Source: CAD feature listing. Evaluate the final solid. Frame: model axes, mm. A direction names the side the tool comes from. Give positions to 0.01 mm unless a question says otherwise; leave off trailing zeros. Write each loop counter-clockwise with the first axis right and the second up, starting at its lowest first coordinate (ties: lowest second). Pieces come first, ordered by that corner, then holes. Notation, with made-up numbers: (38, 4.5) -> (74, 4.5) arc R11 cw to (74, 9.5) -> close; hole circle Ø3 at (30.5, -26). An arc over 180 degrees is marked (long way). Write item = value, one per line.
from build123d import *

# Parameters (mm, degrees)
SKETCH1_W            = 250
SKETCH1_H            = 100
BOSS_EXTRUDE1_DEPTH  = 5
SKETCH2_W            = 5
SKETCH2_H            = 100
BOSS_EXTRUDE2_DEPTH  = 50
FILLET1_R            = 20
BOSS_EXTRUDE3_START  = -250
SKETCH3_R            = 5
BOSS_EXTRUDE3_DEPTH  = 40
BOSS_EXTRUDE4_START  = 40
SKETCH3_2_R          = 5
BOSS_EXTRUDE4_DEPTH  = 40
SKETCH4_R            = 10
BOSS_EXTRUDE5_DEPTH  = 500
SKETCH6_R            = 7.5
BOSS_EXTRUDE9_DEPTH  = 5
BOSS_EXTRUDE11_START = 5
SKETCH7_R            = 7.5
BOSS_EXTRUDE11_DEPTH = 5
FILLET3_R            = 2.5


with BuildPart() as part:
    # Sketch1 → Boss-Extrude1 (new body)
    with BuildSketch(Plane(origin=(0, 0, 0), x_dir=(1, 0, 0), z_dir=(0, 1, 0))):
        Rectangle(SKETCH1_W, SKETCH1_H)
    extrude(amount=BOSS_EXTRUDE1_DEPTH)

    # Sketch2 → Boss-Extrude2 (add)
    with BuildSketch(Plane(origin=(0, 5, 0), x_dir=(1, 0, 0), z_dir=(0, 1, 0))):
        with Locations((-122.5, 0)):
            Rectangle(SKETCH2_W, SKETCH2_H)
        with Locations((122.5, 0)):
            Rectangle(SKETCH2_W, SKETCH2_H)
    extrude(amount=BOSS_EXTRUDE2_DEPTH)

    # Fillet1
    fillet1_edges = [part.edges().sort_by_distance(p)[0] for p in [
        (122.5, 55, -50),
        (122.5, 55, 50),
        (-122.5, 55, -50),
        (-122.5, 55, 50),
    ]]
    fillet(fillet1_edges, radius=FILLET1_R)

    # Sketch3 → Boss-Extrude3 (add)
    with BuildSketch(Plane.ZY.offset(125).offset(BOSS_EXTRUDE3_START)):
        with Locations((0, 27.5)):
            Circle(SKETCH3_R)
    extrude(amount=-BOSS_EXTRUDE3_DEPTH)

    # Sketch3<2> → Boss-Extrude4 (add)
    with BuildSketch(Plane.ZY.offset(125).offset(BOSS_EXTRUDE4_START)):
        with Locations((0, 27.5)):
            Circle(SKETCH3_2_R)
    extrude(amount=-BOSS_EXTRUDE4_DEPTH)

    # Sketch4 → Boss-Extrude5 (add)
    with BuildSketch(Plane(origin=(0, 0, 0), x_dir=(-1, 0, 0), z_dir=(0, -1, 0))):
        with Locations(Location((0, 0, 0), (0, 0, 270))):
            Circle(SKETCH4_R)
    extrude(amount=BOSS_EXTRUDE5_DEPTH)

    # Sketch6 → Boss-Extrude9 (add)
    with BuildSketch(Plane(origin=(165, 0, 0), x_dir=(0, 0, -1), z_dir=(1, 0, 0))):
        with Locations((0, 27.5)):
            Circle(SKETCH6_R)
    extrude(amount=BOSS_EXTRUDE9_DEPTH)

    # Sketch7 → Boss-Extrude11 (add)
    with BuildSketch(Plane.ZY.offset(165).offset(BOSS_EXTRUDE11_START)):
        with Locations(Location((0, 27.5, 0), (0, 0, 180))):
            Circle(SKETCH7_R)
    extrude(amount=-BOSS_EXTRUDE11_DEPTH)

    # Fillet3
    fillet3_edges = [part.edges().sort_by_distance(p)[0] for p in [
        (-120, 5, 0),
        (120, 5, 0),
    ]]
    fillet(fillet3_edges, radius=FILLET3_R)


solid = part.part
(1) Section query D-D (x = -104). Return loops of the section in (y, z), plus the area to 3 significant figures.
Values follow:
outline = (0, -50) -> (5, -50) -> (5, 50) -> (0, 50) -> close
area = 500 mm2
(2) Section query B-B (z = 40). Return loops of the section in (x, y).
Values follow:
outline = (-125, 0) -> (125, 0) -> (125, 52.32) -> (120, 52.32) -> (120, 7.5) arc R2.5 cw to (117.5, 5) -> (-117.5, 5) arc R2.5 cw to (-120, 7.5) -> (-120, 52.32) -> (-125, 52.32) -> close
(3) Section query C-C (y = -123). Return loops of the section in (x, z), plus the area to 3 significant figures.
Values follow:
outline = circle Ø20 at (0, 0)
area = 314 mm2
(4) Access query for faces 1 (the face through (0, -500, 0)), 2 (the face through (-145.28, 22.62, -1.08)), 3 (the face through (122.535, 48.986, 44.297)), 4 (the face through (9.76, -246.5, -2.17)), 5 (the face through (-2, 5, -1)). Directions: +Z, -Z, +X, -X, +Y, -Y. A direction counts if a zero-diameter tool reaches every point of the face in a straight line with its end or side. Return the directions, or none.
Values follow:
face_1 = +Z, -Z, +X, -X, -Y
face_2 = none
face_3 = +Z, +X, -X, +Y
face_4 = -Y
face_5 = +Z, -Z, +Y
(5) Pull-direction query (X, two-part tool) for faces 6 (the face through (-170, 27, 0)), 7 (the face through (120, 31, 1)), 8 (the face through (-2, 0, -12)); classes: pulls with the +X half, pulls with the -X half, needs draft (parallel to the pull), parting line crosses it, or undercut.
Values follow:
face_6 = pulls with the -X half
face_7 = undercut
face_8 = needs draft
(6) Section query A-A (x = 0). Return loops of the section in (y, z), plus the area to 3 significant figures.
Values follow:
outline = (-500, -10) -> (0, -10) -> (0, -50) -> (5, -50) -> (5, 50) -> (0, 50) -> (0, 10) -> (-500, 10) -> close
area = 10,500 mm2
(7) Material intervals for line 1 (Y direction, x = 15, z = 17.5); line 2 (Y direction, x = 118, z = 32); line 3 (X direction, y = -239, z = -6), sorted ascending.
Values follow:
line_1 = 0 to 5
line_2 = 0 to 5.05
line_3 = -8 to 8
(8) First-contact query: pin 1 (6 mm diameter, centred on x = 12, y = -303, fed in from -Z); pin 2 (12 mm diameter, centred on y = -191.5, z = 5, fed in from +X); pin 3 (6 mm diameter, centred on x = -70, z = 4.5, fed in from +Y). Flat tips, straight axial feed; report the tip coordinate or a pass-through.
Values follow:
pin_1 = -4.36
pin_2 = 10
pin_3 = 5
